Here's the drawing with two shaded views (mm, measured from the low corner). I have some questions. Round coordinates to 2 decimals unless told otherwise and drop trailing zeros. Loops run counter-clockwise (first coordinate to the right, second up) from the corner with the lowest first, then second, coordinate; pieces in that order, holes last.
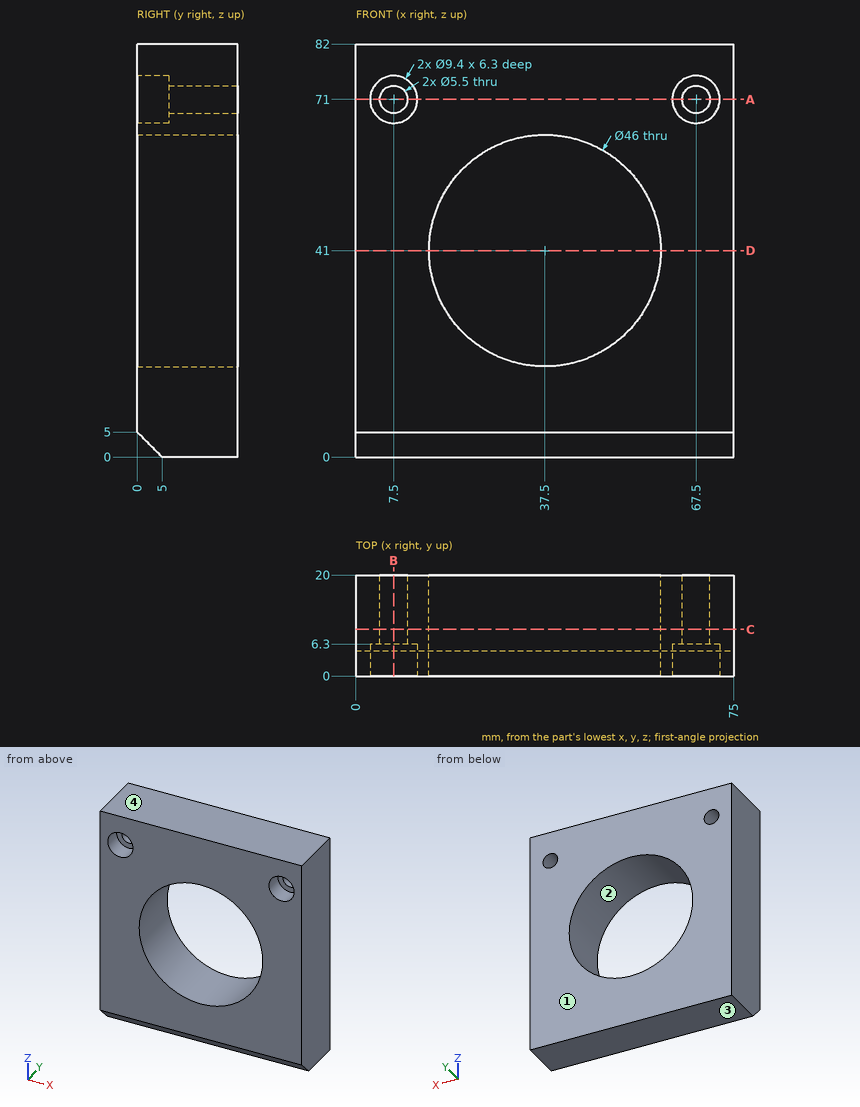
Item 1: Will this pin go through, and if not, where does the flat tip stop? pin 1 (7 mm diameter, centred on x = 7.5, z = 71, fed in from -Y).
Results list:
pin 1: stops at y = 6.3
Item 2: If we section it at B-B, the plane x = 7.5: Please give me the cut outline in (y, z).
Results list:
outline: (0, 5) - (5, 0) - (20, 0) - (20, 68.25) - (6.3, 68.25) - (6.3, 66.3) - (0, 66.3) - close; (0, 75.7) - (6.3, 75.7) - (6.3, 73.75) - (20, 73.75) - (20, 82) - (0, 82) - close
Item 3: We'd pull the mould along Z, two halves only. Please class the marked faces 1, 2, 3 and 4: released by +Z, released by -Z, zero draft, split by the parting line, or undercut.
Results list:
face 1: zero draft
face 2: undercut
face 3: released by -Z
face 4: released by +Z
Item 4: If we section it at A-A, the plane z = 71: Please give me the cut outline in (x, y), then the cut area to 3 significant figures.
Results list:
outline: (0, 0) - (2.8, 0) - (2.8, 6.3) - (4.75, 6.3) - (4.75, 20) - (0, 20) - close; (10.25, 6.3) - (12.2, 6.3) - (12.2, 0) - (62.8, 0) - (62.8, 6.3) - (64.75, 6.3) - (64.75, 20) - (10.25, 20) - close; (70.25, 6.3) - (72.2, 6.3) - (72.2, 0) - (75, 0) - (75, 20) - (70.25, 20) - close
area: 1,230 mm2
Item 5: If we section it at C-C, the plane y = 9.25: Please give me the cut outline in (x, z).
Results list:
outline: (0, 0) - (75, 0) - (75, 82) - (0, 82) - close; hole circle Ø5.5 at (7.5, 71); hole circle Ø46 at (37.5, 41); hole circle Ø5.5 at (67.5, 71)
Item 6: If I drill on line 1 along X through (y, z) = (16.25, 71); line 2 along Z through (x, y) = (37.5, 13); line 3 along X through (y, z) = (18.75, 69.5), over which ranges is the centre line in solid material (lowest first)?
Results list:
line 1: x = 0 to 4.75, 10.25 to 64.75, 70.25 to 75
line 2: z = 0 to 18, 64 to 82
line 3: x = 0 to 5.2, 9.8 to 65.2, 69.8 to 75
Item 7: If we section it at D-D, the plane z = 41: Please give me the cut outline in (x, y), then the cut area to 3 significant figures.
Results list:
outline: (0, 0) - (14.5, 0) - (14.5, 20) - (0, 20) - close; (60.5, 0) - (75, 0) - (75, 20) - (60.5, 20) - close
area: 580 mm2
